```python
from build123d import *

# Parameters (mm, degrees)
F1_R     = 10.9982
F1_R_2   = 14.2875
F2_DEPTH = 6.35
F0_R     = 14.2875
F0_R_2   = 10.9982
F3_DEPTH = 6.35
F4_R     = 2.520905
F5_DEPTH = 6.351


with BuildPart() as f2:
    # F1 (on Front) → F2 (new body)
    with BuildSketch(Plane.XZ):
        with BuildLine():
            ThreePointArc((14.2875, 31.75), (-3.161339, 45.683363), (-12.888506, 25.58404))
            ThreePointArc((-12.888506, 25.58404), (0, 17.4625), (12.888506, 25.58404))
            ThreePointArc((12.888506, 25.58404), (13.933363, 28.588661), (14.2875, 31.75))
        make_face()
        with Locations((0, 31.75)):
            Circle(F1_R, mode=Mode.SUBTRACT)
        with BuildLine():
            ThreePointArc((41.783807, -15.875), (37.982283, -6.170519), (28.600682, -1.630246))
            ThreePointArc((28.600682, -1.630246), (15.122969, -8.73125), (15.712175, -23.953793))
            ThreePointArc((15.712175, -23.953793), (31.725188, -29.522315), (41.783807, -15.875))
        make_face()
        with Locations((27.496307, -15.875)):
            Circle(F1_R, mode=Mode.SUBTRACT)
        with BuildLine():
            ThreePointArc((-13.208807, -15.875), (-17.791826, -5.389023), (-28.600681, -1.630246))
            ThreePointArc((-28.600681, -1.630246), (-39.869645, -23.01875), (-15.712175, -23.953793))
            ThreePointArc((-15.712175, -23.953793), (-13.848991, -20.103882), (-13.208807, -15.875))
        make_face()
        with Locations((-27.496307, -15.875)):
            Circle(F1_R, mode=Mode.SUBTRACT)
        with BuildLine():
            ThreePointArc((-12.888506, 25.58404), (-11.495364, 21.577878), (-11.023181, 17.362759))
            ThreePointArc((-11.023181, 17.362759), (-16.091879, 4.423451), (-28.600681, -1.630246))
            ThreePointArc((-28.600681, -1.630246), (-17.791826, -5.389023), (-13.208807, -15.875))
            ThreePointArc((-13.208807, -15.875), (-13.848991, -20.103882), (-15.712175, -23.953793))
            ThreePointArc((-15.712175, -23.953793), (0, -15.675518), (15.712175, -23.953793))
            ThreePointArc((15.712175, -23.953793), (15.122969, -8.73125), (28.600682, -1.630246))
            ThreePointArc((28.600682, -1.630246), (13.575397, 7.837759), (12.888506, 25.58404))
            ThreePointArc((12.888506, 25.58404), (0, 17.4625), (-12.888506, 25.58404))
        make_face()
        Circle(F1_R_2, mode=Mode.SUBTRACT)
    extrude(amount=F2_DEPTH)

    # F0 (on Front) → F3 (join)
    with BuildSketch(Plane.XZ):
        Circle(F0_R)
        Circle(F0_R_2, mode=Mode.SUBTRACT)
    extrude(amount=F3_DEPTH)

    # F4 (on face) → F5 (cut, through all)
    with BuildSketch(Plane.XZ.offset(6.35)):
        with Locations((0, 15.981898)):
            Circle(F4_R)
        with Locations((-13.840729, -7.990949)):
            Circle(F4_R)
        with Locations((13.840729, -7.990949)):
            Circle(F4_R)
    extrude(amount=-F5_DEPTH, mode=Mode.SUBTRACT)


solid = f2.part
```
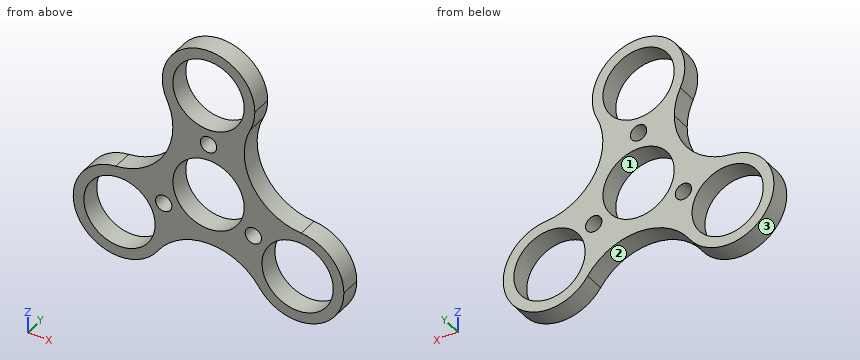
The listing builds one solid part. Answer for the finished solid, in the listing's coordinates (mm). Face numbers are marked on the shaded views. Coordinates: 2 decimals unless noted, no trailing zeros. Loops run counter-clockwise (first coordinate to the right, second up) from the corner with the lowest first, then second, coordinate; pieces in that order, holes last. Notation, with made-up numbers: M 45,31 L 61,31 A23 ccw 61,59 Z; hole C 22.25,-32 d6. An arc over 180 degrees is marked long. Answer as a JSON object with one key per item and string values. Group by question number.
Item 1: Section B-B (z = 33) is taken. Write down the section's boundary in (x, y).
Item 2: Section A-A (x = 0) is taken. Write down the section's boundary in (y, z), and give its area (3 significant figures).
Item 3: Consider L1, parallel to Z at x = 0, y = -2; L2, parallel to Z at x = -1, y = -4.25; L3, parallel to X at y = -4.75, z = -21.5. Determine where each line is inside the solid, lowest interval first.
Item 4: Determine the mould class of the marked faces 1, 2 and 3 for opening direction Z: +Z half, -Z half, draft (parallel to the pull), parting line (faces both ways), or undercut.
Item 5: Each of these flat-tipped pins is pushed along its axis until it touches: P1, Ø3, axis at y = -1.5, z = 19.5, coming from the -X side; P2, Ø4, axis at x = 13.84, z = -7.99, coming from the +Y side; P3, Ø3, axis at x = 21.5, y = -3.5, coming from the +Z side; P4, Ø2, axis at x = -32.5, y = -5, coming from the +Z side. Where does it stop, or does it pass through?
Item 6: Section D-D (y = -4.5) is taken. Give the number of separate pieces and of enclosed holes in the cut face, and give its area (3 significant figures).
Item 7: Section C-C (x = 19) is taken. Write down the section's boundary in (y, z).
Solved:
{
 "1": {"outline": "M -14.23,-6.35 L -10.93,-6.35 L -10.93,0 L -14.23,0 Z; M 10.93,-6.35 L 14.23,-6.35 L 14.23,0 L 10.93,0 Z"},
 "2": {"outline": "M -6.35,-15.68 L 0,-15.68 L 0,-11 L -6.35,-11 Z; M -6.35,11 L 0,11 L 0,13.46 L -6.35,13.46 Z; M -6.35,18.5 L 0,18.5 L 0,20.75 L -6.35,20.75 Z; M -6.35,42.75 L 0,42.75 L 0,46.04 L -6.35,46.04 Z", "area": "80.5 mm2"},
 "3": {"L1": "z = -15.68 to -11, 11 to 13.46, 18.5 to 20.75, 42.75 to 46.04", "L2": "z = -15.7 to -10.95, 10.95 to 13.67, 18.3 to 20.8, 42.7 to 46", "L3": "x = -40.63 to -36.95, -18.05 to -13.71, 13.71 to 18.05, 36.95 to 40.63"},
 "4": {"face 1": "undercut", "face 2": "-Z half", "face 3": "parting line"},
 "5": {"P1": "stops at x = -11.37", "P2": "passes through", "P3": "stops at z = 1.19", "P4": "stops at z = -2.16"},
 "6": {"separate pieces": "1", "enclosed holes": "7", "area": "1,460 mm2"},
 "7": {"outline": "M -6.35,-27.36 L 0,-27.36 L 0,-22.86 L -6.35,-22.86 Z; M -6.35,-8.89 L 0,-8.89 L 0,1.86 L -6.35,1.86 Z"}
}
